```python
from build123d import *

# Parameters (mm, degrees)
ESQUISSE1_W        = 88.328603511
ESQUISSE1_H        = 74.903508165
BOSS_EXTRU_1_DEPTH = 3
D_GAGEMENT_M31_D   = 3.4


with BuildPart() as part:
    # Esquisse1 → Boss.-Extru.1 (new body)
    with BuildSketch(Plane.XY):
        with Locations((-13.227677397, -0.159821294)):
            Rectangle(ESQUISSE1_W, ESQUISSE1_H)
    extrude(amount=-BOSS_EXTRU_1_DEPTH)

    # Dégagement M31 (through all)
    with Locations(Plane.XY):
        with Locations((26.095, 8.89), (-24.825, 24.13), (-26.095, -24.13)):
            Hole(D_GAGEMENT_M31_D / 2)


solid = part.part
```
Input: part model. Units: mm. Frame: model coordinates. Give positions to 0.01 mm unless a question says otherwise; leave off trailing zeros. Order: outer loops, then holes, each group sorted by start corner. A loop starts at its lowest first (then second) coordinate and runs counter-clockwise, first axis right, second up. Notation, with made-up numbers: (53, 77) - (111, 77) arc R36 ccw to (111, 113) - close; hole circle Ø10 at (79.5, 58.5). An arc over 180 degrees is marked (long way). Put each result on its own line as item: value.
Item 1: Ray query, L1, parallel to Y at x = -26, z = -1. Return the intervals inside material, ascending. Write a range as from..to.
Found:
L1: y = -37.61..-25.83, -22.43..22.9, 25.36..37.29
Item 2: Section query A-A, the plane y = -24.13. Return loops of the section in (x, z) (3 decimals).
Found:
outline: (-57.392, -3) - (-27.795, -3) - (-27.795, 0) - (-57.392, 0) - close; (-24.395, -3) - (30.937, -3) - (30.937, 0) - (-24.395, 0) - close
Item 3: Contact query for a flat-ended pin moving along its axis: pin 1 (4.5 mm diameter, centred on x = 26.095, y = 8.89, fed in from -Z). Output: stop coordinate, or through.
Found:
pin 1: stops at z = -3
Item 4: Draft query along Y for faces 1 (the cylindrical face through (-26.88, -25.64, -1.52)), 2 (the flat face through (-14, 0, 0)), 3 (the flat face through (-14, -37.612, -1)). Return one class per face: +Y half, -Y half, draft (parallel to the pull), parting line (faces both ways), or undercut.
Found:
face 1: undercut
face 2: draft
face 3: -Y half
